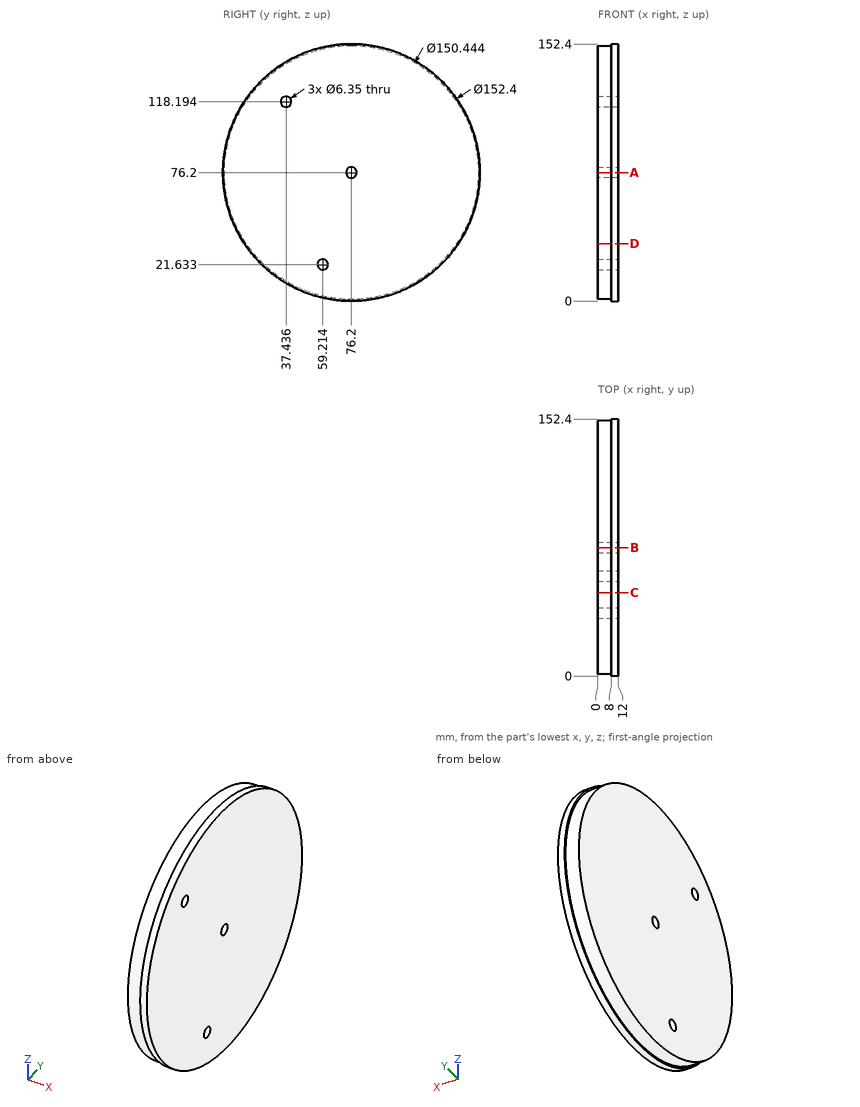
Print and shaded views of the part. All mm, measured from the part's lowest x, y and z. Give positions to 0.01 mm unless a question says otherwise; leave off trailing zeros. Loops run counter-clockwise (first coordinate to the right, second up) from the corner with the lowest first, then second, coordinate; pieces in that order, holes last. Notation, with made-up numbers: (51.25, 65) -> (65.25, 65) arc R23 ccw to (65.25, 76) -> close; hole circle Ø10 at (48, -23.75). An arc over 180 degrees is marked (long way). Answer in a Markdown table with one row per item.
Item 1: Slice it at D-D on z = 34. Write the cut outline in (x, y).
Findings below:
| item | result |
|---|---|
| outline | (0, 13.93) -> (8, 13.93) -> (8, 12.75) -> (12, 12.75) -> (12, 139.65) -> (8, 139.65) -> (8, 138.47) -> (0, 138.47) -> close |
Item 2: Slice it at C-C on y = 49.5. Write the cut outline in (x, z).
Findings below:
| item | result |
|---|---|
| outline | (0, 5.88) -> (8, 5.88) -> (8, 4.83) -> (12, 4.83) -> (12, 147.57) -> (8, 147.57) -> (8, 146.52) -> (0, 146.52) -> close |
Item 3: Probe line 1 along Y through (x, z) = (4.5, 76.2) (1 decimal); line 2 along Y through (x, z) = (9, 76.2) (1 decimal); line 3 along Z through (x, y) = (9, 74). List the from-to ranges inside material, lowest first. Write a range as [from, to].
Findings below:
| item | result |
|---|---|
| line 1 | y = [1, 73], [79.4, 151.4] |
| line 2 | y = [0, 73], [79.4, 152.4] |
| line 3 | z = [0.03, 73.91], [78.49, 152.37] |
Item 4: Slice it at A-A on z = 76.2. Write the cut outline in (x, y) (1 decimal), plus the area to 3 significant figures.
Findings below:
| item | result |
|---|---|
| outline | (0, 1) -> (8, 1) -> (8, 0) -> (12, 0) -> (12, 73) -> (0, 73) -> close; (0, 79.4) -> (12, 79.4) -> (12, 152.4) -> (8, 152.4) -> (8, 151.4) -> (0, 151.4) -> close |
| area | 1,740 mm² |
Item 5: Flat gauge pins, fed straight in: P1, Ø5, axis at x = 7, y = 102, coming from the +Z side; P2, Ø6, axis at x = 2.5, y = 33, coming from the -Z side; P3, Ø4, axis at x = 7.5, y = 136.5, coming from the -Z side. Where does each tip first touch, or does it go through?
Findings below:
| item | result |
|---|---|
| P1 | stops at z = 148.68 |
| P2 | stops at z = 12.62 |
| P3 | stops at z = 27.21 |
